Source: three-view drawing plus pictorial views. Frame: mm from the lowest corner of the part. A direction names the side the tool comes from. Coordinates: 2 decimals unless noted, no trailing zeros. Loops run counter-clockwise (first coordinate to the right, second up) from the corner with the lowest first, then second, coordinate; pieces in that order, holes last.
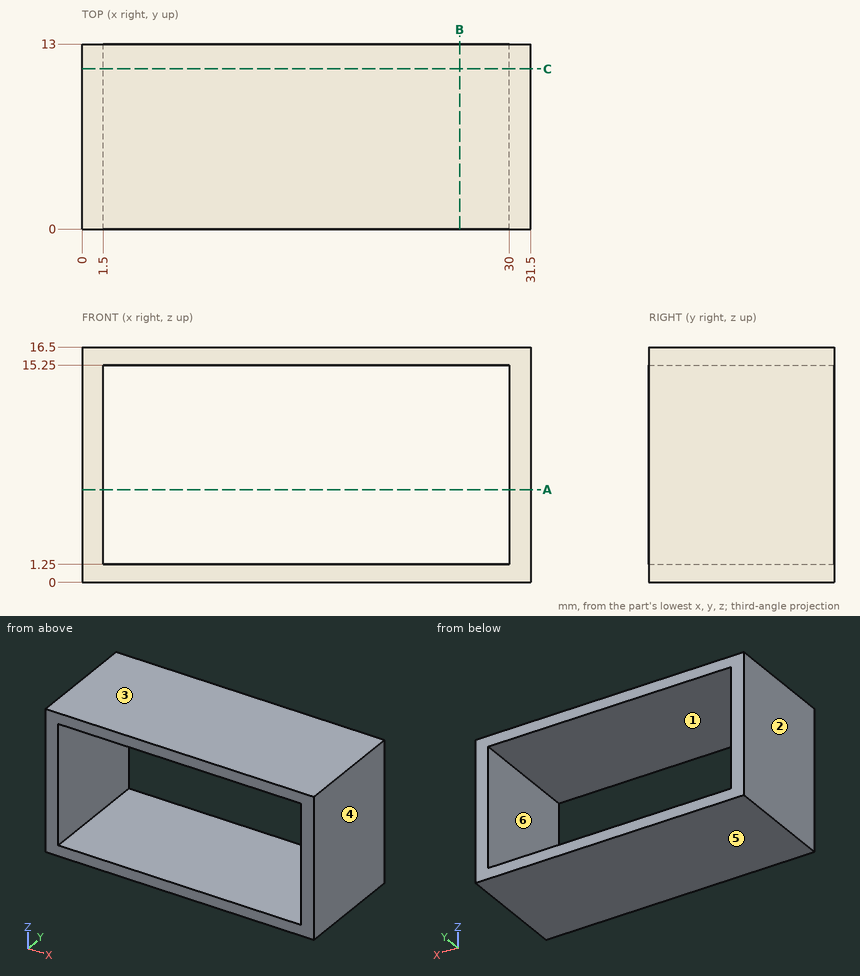
Q1. Draft query along X for the marked faces 1, 2, 3 and 4. Return one class per face: released by +X, released by -X, zero draft, split by the parting line, or undercut.
Q2. Section query B-B on x = 26.5. Return the cut outline in (y, z), then the cut area to 3 significant figures.
Q3. Section query A-A on z = 6.5. Return the cut outline in (x, y).
Q4. Material intervals for line 1 along Z through (x, y) = (6.5, 9.75); line 2 along X through (y, z) = (8, 10.25), sorted ascending.
Q5. Section query C-C on y = 11.25. Return the cut outline in (x, z).
Q6. First-contact query: pin 1 Ø2 at (x, y) = (17, 8) entering from -Z. Flat tip, straight axial feed; report the tip coordinate or a pass-through.
Q7. Reachability of the marked faces 5 and 6 from +Z, -Z, +X, -X, +Y, -Y: full face, straight path, thin tool, end or side. Return the list, or none.
Resolved:
1. face 1: undercut
1. face 2: released by -X
1. face 3: zero draft
1. face 4: released by +X
2. outline: (0, 0) - (13, 0) - (13, 1.25) - (0, 1.25) - close; (0, 15.25) - (13, 15.25) - (13, 16.5) - (0, 16.5) - close
2. area: 32.5 mm2
3. outline: (0, 0) - (1.5, 0) - (1.5, 13) - (0, 13) - close; (30, 0) - (31.5, 0) - (31.5, 13) - (30, 13) - close
4. line 1: z = 0 to 1.25, 15.25 to 16.5
4. line 2: x = 0 to 1.5, 30 to 31.5
5. outline: (0, 0) - (31.5, 0) - (31.5, 16.5) - (0, 16.5) - close; hole (1.5, 1.25) - (30, 1.25) - (30, 15.25) - (1.5, 15.25) - close
6. pin 1: stops at z = 0
7. face 5: -Z, +X, -X, +Y, -Y
7. face 6: +Y, -Y
